from build123d import *

# Parameters (mm, degrees)
SKETCH1_R           = 4.445
SKETCH1_R_2         = 3.275000003
BOSS_EXTRUDE1_DEPTH = 10.16
SKETCH2_W           = 8.89
SKETCH2_H           = 8.89
BOSS_EXTRUDE2_DEPTH = 25.4
BOSS_EXTRUDE3_REACH = 29.275
SKETCH9_R           = 2.2499955
CUT_EXTRUDE1_DEPTH  = 30.863820986
SKETCH11_R          = 2.2499955
CUT_EXTRUDE4_DEPTH  = 6.38999992


with BuildPart() as part:
    # Sketch1 → Boss-Extrude1 (new body)
    with BuildSketch(Plane.XY):
        Circle(SKETCH1_R)
        Circle(SKETCH1_R_2, mode=Mode.SUBTRACT)
    extrude(amount=BOSS_EXTRUDE1_DEPTH)

    # Sketch2 → Boss-Extrude2 (add)
    with BuildSketch(Plane(origin=(0, 0, 0), x_dir=(-1, 0, 0), z_dir=(0, 0, -1))):
        Rectangle(SKETCH2_W, SKETCH2_H)
    extrude(amount=BOSS_EXTRUDE2_DEPTH)

    # Boss-Extrude3: up to this face of the body (flat: up to its plane)
    boss_extrude3_end = Plane(part.part.faces().sort_by_distance((0, 4.445, -12.7))[0])
    # Sketch8 → Boss-Extrude3 (add, up to the picked face)
    with BuildSketch(Plane(origin=(0, -4.445, 0), x_dir=(-1, 0, 0), z_dir=(0, -1, 0)), mode=Mode.PRIVATE) as boss_extrude3_sk1:
        with BuildLine():
            Line((7.784941034, 19.641513294), (4.445, 0))
            Line((4.445, 0), (-4.445, 0))
            Line((-4.445, 0), (-7.784941034, 19.641513294))
            ThreePointArc((-7.784941034, 19.641513294), (0, 27.426454328), (7.784941034, 19.641513294))
        make_face()
    boss_extrude3_tool1 = split(extrude(boss_extrude3_sk1.sketch, amount=-BOSS_EXTRUDE3_REACH, mode=Mode.PRIVATE), bisect_by=boss_extrude3_end, keep=Keep.BOTH, mode=Mode.PRIVATE)
    add(boss_extrude3_tool1.solids().sort_by(Axis((0, -4.445, -14.186159), (0, 1, 0)))[0])

    # Sketch9 → Cut-Extrude1 (cut, through all)
    with BuildSketch(Plane(origin=(0, 4.445, 0), x_dir=(1, 0, 0), z_dir=(0, 1, 0))):
        with Locations(Location((0, 19.853346126, 0), (0, 0, 180))):
            Circle(SKETCH9_R)
    extrude(amount=-CUT_EXTRUDE1_DEPTH, mode=Mode.SUBTRACT)

    # Sketch11 → Cut-Extrude4 (cut)
    with BuildSketch(Plane.XZ.offset(4.445)):
        with BuildLine():
            Line((5.521223684, -6.329052393), (-5.521223684, -6.329052393))
            Line((-5.521223684, -6.329052393), (-7.784941034, -19.641513294))
            ThreePointArc((-7.784941034, -19.641513294), (0, -27.426454328), (7.784941034, -19.641513294))
            Line((7.784941034, -19.641513294), (5.521223684, -6.329052393))
        make_face()
        with Locations(Location((0, -19.853346126, 0), (0, 0, 180))):
            Circle(SKETCH11_R, mode=Mode.SUBTRACT)
    extrude(amount=-CUT_EXTRUDE4_DEPTH, mode=Mode.SUBTRACT)


solid = part.part
Verification items for the finished model (mm, model axes). A direction names the side the tool comes from. Round coordinates to 2 decimals unless told otherwise and drop trailing zeros. Loops run counter-clockwise (first coordinate to the right, second up) from the corner with the lowest first, then second, coordinate; pieces in that order, holes last. Notation, with made-up numbers: M 33.5,1.5 L 55.5,1.5 A7 cw 55.5,14.5 Z; hole C -36.75,2 d9. An arc over 180 degrees is marked long. Write each question's results on one line, items separated by ' | '.
1) Section check D-D on z = -11.5. Record the boundary of the cut face in (x, y) (3 decimals).
Checks:
outline: M -6.401,1.945 L 6.401,1.945 L 6.401,4.445 L -6.401,4.445 Z
2) Section check B-B on y = 1. Record the boundary of the cut face in (x, z) (3 decimals), then the cut area to 3 significant figures.
Checks:
outline: M -5.521,-6.329 L 5.521,-6.329 L 4.445,0 L 4.331,0 L 4.331,10.16 L 3.119,10.16 L 3.119,0 L -3.119,0 L -3.119,10.16 L -4.331,10.16 L -4.331,0 L -4.445,0 Z | area: 87.7 mm2
3) Mould release check, pull along X, two halves, no side actions. Record for faces 1 (the flat face through (-2, -3, 10.16)), 2 (the cylindrical face through (0.171, 3.177, -27.425)), 3 (the cylindrical face through (-2.6, -1.99, 5.01)): released by +X, released by -X, zero draft, split by the parting line, or undercut.
Checks:
face 1: zero draft | face 2: split by the parting line | face 3: undercut
4) Gauge pin test, flat ends, axial feed: P1, Ø3.5, axis at x = 1, y = 0, coming from the +Z side; P2, Ø5, axis at x = 3.5, y = 1, coming from the -Z side; P3, Ø3, axis at x = 0.5, y = -1, coming from the -Z side. Record the tip position at first contact, or that the pin passes through.
Checks:
P1: stops at z = 0 | P2: stops at z = -27.34 | P3: stops at z = -6.33
5) Scan lines: L1, parallel to Z at x = 0, y = 3.85; L2, parallel to X at y = 2, z = -20; L3, parallel to Z at x = 0, y = 2.7. Record each from-to range of solid material in increasing order. Write a range as from..to.
Checks:
L1: z = -27.43..-22.1, -17.6..10.16 | L2: x = -7.78..-2.25, 2.25..7.78 | L3: z = -27.43..-22.1, -17.6..0
6) Access from +Z, -Z, +X, -X, +Y, -Y to the whole of each face (thin tool, end or side, straight path). Record for faces 4 (the flat face through (4, 3, 0)), 5 (the flat face through (0, -1, -6.329)), 6 (the flat face through (4, -3, 0)).
Checks:
face 4: +Z, +X, +Y | face 5: -Z, +X, -X, -Y | face 6: +Z, +X, -Y
7) Section check C-C on x = -6.5. Record the boundary of the cut face in (y, z) (3 decimals).
Checks:
outline: M 1.945,-23.926 L 4.445,-23.926 L 4.445,-12.085 L 1.945,-12.085 Z
8) Section check A-A on y = 2.5. Record the boundary of the cut face in (x, z) (3 decimals), then the cut area to 3 significant figures.
Checks:
outline: M -7.785,-19.642 A7.785 ccw 7.785,-19.642 L 4.445,0 L 3.675,0 L 3.675,10.16 L 2.116,10.16 L 2.116,0 L -2.116,0 L -2.116,10.16 L -3.675,10.16 L -3.675,0 L -4.445,0 Z; hole C 0,-19.853 d4.5 | area: 351 mm2
